Check sheet for the modelled part. Datum: model origin and axes. Units: mm. Give positions to 0.01 mm unless a question says otherwise; leave off trailing zeros. Order: outer loops, then holes, each group sorted by start corner. A loop starts at its lowest first (then second) coordinate and runs counter-clockwise, first axis right, second up.
Item 1: Sectioned sample at B-B on x = 397. Record the boundary of the cut face in (y, z), and give its area (3 significant figures).
Item 2: Sectioned sample at A-A on y = -124.5. Record the boundary of the cut face in (x, z).
Item 3: Sectioned sample at D-D on x = -28. Record the boundary of the cut face in (y, z), and give its area (3 significant figures).
Item 4: Gauge pin test, flat ends, axial feed: P1, Ø4, axis at x = -149, y = 1.5, coming from the -Z side; P2, Ø3, axis at x = -142, z = 6.5, coming from the -Y side; P3, Ø4, axis at y = -19, z = 7.5, coming from the +X side; P4, Ø1.5, axis at y = 127, z = 8.5, coming from the +X side. Record the tip position at first contact, or that the pin passes through.
Item 5: Sectioned sample at C-C on z = 7.75. Count the separate pieces of the cut face and the enclosed holes in it, and give its area (3 significant figures).
Item 6: Material ranges on line 1 along X through (y, z) = (-27, 9.75); line 2 along X through (y, z) = (-92, 6); line 3 along Y through (x, z) = (362.5, 8.25), recorded low to high.
from build123d import *

# Parameters (mm, degrees)
BOSS_EXTRUDE1_DEPTH = 10
CUT_EXTRUDE1_DEPTH  = 10
CUT_EXTRUDE2_DEPTH  = 10


with BuildPart() as part:
    # Sketch2 → Boss-Extrude1 (new body)
    with BuildSketch(Plane.XY):
        with BuildLine():
            Line((-257, -160), (-126.694416638, -70.567832456))
            Line((-126.694416638, -70.567832456), (126.694416638, -70.567832456))
            Line((126.694416638, -70.567832456), (257, -160))
            Line((257, -160), (457, -160))
            Line((457, -160), (457, 47.365686012))
            Line((457, 47.365686012), (489.618964007, 120.413637298))
            ThreePointArc((489.618964007, 120.413637298), (489.82769414, 128.064459181), (484.565340597, 133.622001709))
            Line((484.565340597, 133.622001709), (297.41734098, 217.19140723))
            ThreePointArc((297.41734098, 217.19140723), (289.766519097, 217.400137363), (284.208976569, 212.13778382))
            Line((284.208976569, 212.13778382), (253.339865194, 143.008508485))
            Line((253.339865194, 143.008508485), (-232, 143.008508485))
            Line((-232, 143.008508485), (-260.982148435, 229.584058556))
            ThreePointArc((-260.982148435, 229.584058556), (-266.004269265, 235.359605814), (-273.639373591, 235.892358751))
            Line((-273.639373591, 235.892358751), (-479.673848241, 166.919978879))
            ThreePointArc((-479.673848241, 166.919978879), (-485.449395499, 161.897858049), (-485.982148435, 154.262753723))
            Line((-485.982148435, 154.262753723), (-457, 67.687203652))
            Line((-457, 67.687203652), (-457, -160))
            Line((-457, -160), (-257, -160))
        make_face()
    extrude(amount=BOSS_EXTRUDE1_DEPTH)

    # Sketch3 → Cut-Extrude1 (cut)
    with BuildSketch(Plane.XY.offset(10)):
        with BuildLine():
            Line((-456.568069909, 138.128067643), (-447.737597005, 109.744404736))
            ThreePointArc((-447.737597005, 109.744404736), (-442.025570712, 102.884114481), (-433.135600426, 102.072169246))
            Line((-433.135600426, 102.072169246), (-272.142751839, 152.15883325))
            ThreePointArc((-272.142751839, 152.15883325), (-265.282461584, 157.870859543), (-264.470516349, 166.760829829))
            Line((-264.470516349, 166.760829829), (-273.300989253, 195.144492736))
            ThreePointArc((-273.300989253, 195.144492736), (-279.013015546, 202.004782992), (-287.902985832, 202.816728227))
            Line((-287.902985832, 202.816728227), (-448.895834419, 152.730064222))
            ThreePointArc((-448.895834419, 152.730064222), (-455.756124674, 147.01803793), (-456.568069909, 138.128067643))
        make_face()
    extrude(amount=-CUT_EXTRUDE1_DEPTH, mode=Mode.SUBTRACT)

    # Sketch4 → Cut-Extrude2 (cut)
    with BuildSketch(Plane.XY.offset(10)):
        with BuildLine():
            Line((294.889717658, 183.505126769), (282.667716754, 154.360355381))
            ThreePointArc((282.667716754, 154.360355381), (282.628613497, 145.433469155), (288.913225104, 139.093557192))
            Line((288.913225104, 139.093557192), (426.679323763, 81.320677109))
            ThreePointArc((426.679323763, 81.320677109), (435.606209989, 81.281573852), (441.946121952, 87.566185459))
            Line((441.946121952, 87.566185459), (454.168122857, 116.710956847))
            ThreePointArc((454.168122857, 116.710956847), (454.207226114, 125.637843073), (447.922614507, 131.977755036))
            Line((447.922614507, 131.977755036), (310.156515848, 189.750635119))
            ThreePointArc((310.156515848, 189.750635119), (301.229629622, 189.789738376), (294.889717658, 183.505126769))
        make_face()
    extrude(amount=-CUT_EXTRUDE2_DEPTH, mode=Mode.SUBTRACT)


solid = part.part
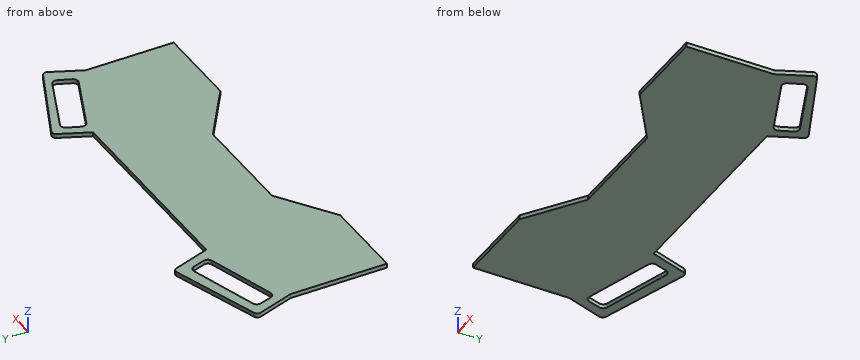
Report:
1. outline: (-160, 0) - (93.77, 0) - (93.77, 10) - (-160, 10) - close; (153.33, 0) - (172.72, 0) - (172.72, 10) - (153.33, 10) - close
1. area: 2,730 mm2
2. outline: (-457, 0) - (-205.28, 0) - (-205.28, 10) - (-457, 10) - close; (205.28, 0) - (457, 0) - (457, 10) - (205.28, 10) - close
3. outline: (-70.57, 0) - (143.01, 0) - (143.01, 10) - (-70.57, 10) - close
3. area: 2,140 mm2
4. P1: stops at z = 0
4. P2: stops at y = -82.1
4. P3: stops at x = 457
4. P4: stops at x = 490.33
5. separate pieces: 1
5. enclosed holes: 2
5. area: 249,000 mm2
6. line 1: x = -457 to 457
6. line 2: x = -457 to -157.92, 157.92 to 457
6. line 3: y = -160 to 108.23, 167.8 to 188.13
